```python
from build123d import *

# Parameters (mm, degrees)
F0_W     = 67
F0_H     = 150
F2_DEPTH = 32
F3_R     = 34
F4_DEPTH = 32
F1_R     = 12
F5_DEPTH = 15


with BuildPart() as f2:
    # F0 (on Top) → F2 (new body)
    with BuildSketch(Plane.XY):
        with Locations((-38.256745, -75)):
            Rectangle(F0_W, F0_H)
    extrude(amount=F2_DEPTH)

    # F3 (on face) → F4 (cut)
    with BuildSketch(Plane.XY.offset(32)):
        with Locations((-71.756745, -75)):
            Circle(F3_R)
    extrude(amount=-F4_DEPTH, mode=Mode.SUBTRACT)

    # F1 (on face) → F5 (cut)
    with BuildSketch(Plane.XY):
        with Locations((-24.756745, -20)):
            Circle(F1_R)
        with Locations((-24.756745, -130)):
            Circle(F1_R)
    extrude(amount=F5_DEPTH, mode=Mode.SUBTRACT)


solid = f2.part
```
Geometry check sheet. Reference: the model listing, model coordinates, mm. A direction names the side the tool comes from. Give positions to 0.01 mm unless a question says otherwise; leave off trailing zeros. Write each loop counter-clockwise with the first axis right and the second up, starting at its lowest first coordinate (ties: lowest second). Pieces come first, ordered by that corner, then holes. Notation, with made-up numbers: (85, 73.5) -> (115, 73.5) arc R11 cw to (115, 93.5) -> close; hole circle Ø1 at (-15, -13.5). An arc over 180 degrees is marked (long way). One line per question, with ' | ' between items.
Item 1: Depth check by flat-ended pin: pin 1 (12 mm diameter, centred on x = -19, y = -21, fed in from -Z); pin 2 (5 mm diameter, centred on y = -59.5, z = 26.5, fed in from -X); pin 3 (3 mm diameter, centred on y = -47.5, z = 28, fed in from -X). Enter the tip coordinate at first touch or a pass-through.
Determined:
pin 1: z = 15 | pin 2: x = -42.91 | pin 3: x = -54.01
Item 2: Scan lines: line 1 along Y through (x, z) = (-19.5, 12); line 2 along Y through (x, z) = (-22.5, 7.5); line 3 along Y through (x, z) = (-55, 6). Record each from-to range of solid material in increasing order.
Determined:
line 1: -150 to -140.79, -119.21 to -30.79, -9.21 to 0 | line 2: -150 to -141.79, -118.21 to -31.79, -8.21 to 0 | line 3: -150 to -104.58, -45.42 to 0
Item 3: Sectioned sample at C-C, the plane y = -130. Record the boundary of the cut face in (x, z).
Determined:
outline: (-71.76, 0) -> (-36.76, 0) -> (-36.76, 15) -> (-12.76, 15) -> (-12.76, 0) -> (-4.76, 0) -> (-4.76, 32) -> (-71.76, 32) -> close
Item 4: Sectioned sample at B-B, the plane x = -64. Record the boundary of the cut face in (y, z).
Determined:
outline: (-150, 0) -> (-108.1, 0) -> (-108.1, 32) -> (-150, 32) -> close; (-41.9, 0) -> (0, 0) -> (0, 32) -> (-41.9, 32) -> close
Item 5: Access from +Z, -Z, +X, -X, +Y, -Y to the whole of each face (thin tool, end or side, straight path). Record for faces 1 (the flat face through (-4.757, -76, 16)), 2 (the flat face through (-25, -20, 15)).
Determined:
face 1: +Z, -Z, +X, +Y, -Y | face 2: -Z
Item 6: Sectioned sample at A-A, the plane z = 12.5. Record the boundary of the cut face in (x, y), plus the area to 3 significant figures.
Determined:
outline: (-71.76, -150) -> (-4.76, -150) -> (-4.76, 0) -> (-71.76, 0) -> (-71.76, -41) arc R34 cw to (-71.76, -109) -> close; hole circle Ø24 at (-24.76, -130); hole circle Ø24 at (-24.76, -20) | area: 7,330 mm^2
Item 7: Sectioned sample at D-D, the plane z = 23.5. Record the boundary of the cut face in (x, y).
Determined:
outline: (-71.76, -150) -> (-4.76, -150) -> (-4.76, 0) -> (-71.76, 0) -> (-71.76, -41) arc R34 cw to (-71.76, -109) -> close
